```python
from build123d import *

# Parameters (mm, degrees)
EXTRUDE_1_DEPTH     = 10
SKETCH_3_W          = 10
SKETCH_3_H          = 20
EXTRUDE_2_DEPTH     = 15
EXTRUDE_3_DEPTH     = 10
EXTRUDE_4_DEPTH     = 10
SKETCH_6_W          = 10
SKETCH_6_H          = 20
EXTRUDE_5_DEPTH     = 180
SKETCH_7_W          = 10.379175533
SKETCH_7_H          = 10.878140119
SKETCH_7_W_2        = 7.174479062
SKETCH_7_H_2        = 11.599196825
CUT_EXTRUDE_1_DEPTH = 211
SKETCH_8_W          = 5
SKETCH_8_H          = 20
CUT_EXTRUDE_2_DEPTH = 25
SKETCH_9_W          = 6
SKETCH_9_H          = 16
EXTRUDE_6_DEPTH     = 10


with BuildPart() as part:
    # 草图2 → 凸台-拉伸1 (new body)
    with BuildSketch(Plane(origin=(0, 0, 0), x_dir=(1, 0, 0), z_dir=(0, 1, 0))):
        with BuildLine():
            Line((-7, 23), (7, 23))
            ThreePointArc((7, 23), (23.263455967, 16.263455967), (30, 0))
            Line((30, 0), (34, 0))
            ThreePointArc((34, 0), (26.091883092, 19.091883092), (7, 27))
            Line((7, 27), (-7, 27))
            ThreePointArc((-7, 27), (-26.091883092, 19.091883092), (-34, 0))
            Line((-34, 0), (-30, 0))
            ThreePointArc((-30, 0), (-23.263455967, 16.263455967), (-7, 23))
        make_face()
    extrude(amount=EXTRUDE_1_DEPTH)

    # 草图3 → 凸台-拉伸2 (add, symmetric)
    with BuildSketch(Plane(origin=(0, 10, 0), x_dir=(1, 0, 0), z_dir=(0, 1, 0))):
        with Locations((-35, 0)):
            Rectangle(SKETCH_3_W, SKETCH_3_H)
        with Locations((35, 0)):
            Rectangle(SKETCH_3_W, SKETCH_3_H)
    extrude(amount=EXTRUDE_2_DEPTH, both=True)

    # 草图4 → 凸台-拉伸3 (add)
    with BuildSketch(Plane(origin=(40, 0, 0), x_dir=(0, 0, -1), z_dir=(1, 0, 0))):
        with BuildLine():
            Line((-2, -5), (2, -5))
            Line((2, -5), (2, -11))
            ThreePointArc((2, -11), (0, -13), (-2, -11))
            Line((-2, -11), (-2, -5))
        make_face()
    extrude(amount=-EXTRUDE_3_DEPTH)

    # 草图5 → 凸台-拉伸4 (add)
    with BuildSketch(Plane.ZY.offset(40)):
        with BuildLine():
            Line((-2, -5), (2, -5))
            Line((2, -5), (2, -11))
            ThreePointArc((2, -11), (0, -13), (-2, -11))
            Line((-2, -11), (-2, -5))
        make_face()
    extrude(amount=-EXTRUDE_4_DEPTH)

    # 草图6 → 凸台-拉伸5 (add)
    with BuildSketch(Plane(origin=(0, 25, 0), x_dir=(1, 0, 0), z_dir=(0, 1, 0))):
        with Locations((-35, 0)):
            Rectangle(SKETCH_6_W, SKETCH_6_H)
        with Locations((35, 0)):
            Rectangle(SKETCH_6_W, SKETCH_6_H)
    extrude(amount=EXTRUDE_5_DEPTH)

    # 草图7 → 切除-拉伸1 (cut, through all)
    with BuildSketch(Plane.XZ.offset(5)):
        with Locations((-35.189587767, -15.43907006)):
            Rectangle(SKETCH_7_W, SKETCH_7_H)
        with Locations((33.587239531, -15.799598412)):
            Rectangle(SKETCH_7_W_2, SKETCH_7_H_2)
    extrude(amount=-CUT_EXTRUDE_1_DEPTH, mode=Mode.SUBTRACT)

    # 草图8 → 切除-拉伸2 (cut, symmetric)
    with BuildSketch(Plane.XZ.offset(5)):
        with Locations((-37.5, 0)):
            Rectangle(SKETCH_8_W, SKETCH_8_H)
        with Locations((37.5, 0)):
            Rectangle(SKETCH_8_W, SKETCH_8_H)
    extrude(amount=CUT_EXTRUDE_2_DEPTH, both=True, mode=Mode.SUBTRACT)

    # 草图9 → 凸台-拉伸6 (add)
    with BuildSketch(Plane.XY.offset(10)):
        with Locations((43, 28)):
            Rectangle(SKETCH_9_W, SKETCH_9_H)
        with Locations((-43, 28)):
            Rectangle(SKETCH_9_W, SKETCH_9_H)
    extrude(amount=-EXTRUDE_6_DEPTH)


solid = part.part
```
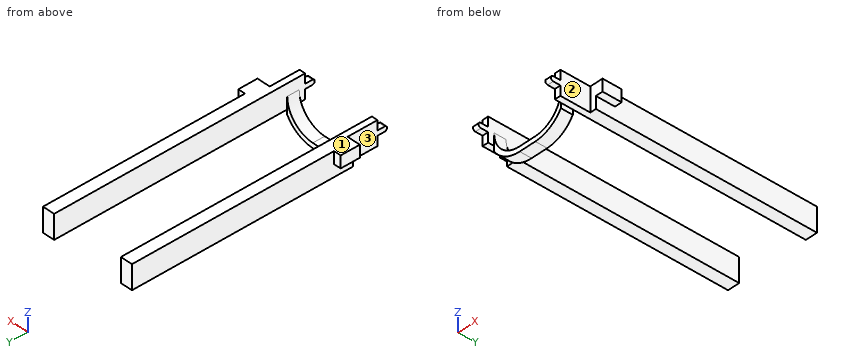
For this review, take the finished solid that the model builds, in its own axes (mm). Face numbers are marked on the shaded views. A direction names the side the tool comes from. Round coordinates to 2 decimals unless told otherwise and drop trailing zeros. Write each loop counter-clockwise with the first axis right and the second up, starting at its lowest first coordinate (ties: lowest second). Pieces come first, ordered by that corner, then holes. Notation, with made-up numbers: (65.25, 78.5) - (101.25, 78.5) arc R19 cw to (101.25, 82.5) - close; hole circle Ø9 at (69, 15.25). An arc over 180 degrees is marked (long way). Answer as CSV lines item,"result". Start each with the question number.
(1) Machinability: for the marked faces 1, 2 and 3, which of the approach directions +Z, -Z, +X, -X, +Y, -Y give a long, thin tool a straight path to every point of the face, cutting with its end or side? Answer none if there is none.
(2) For line 1 (X direction, y = 136.5, z = 8.5); line 2 (X direction, y = 25.5, z = 2); line 3 (Z direction, x = 32, y = 171), list the stretches that pass through material, from the lowest coordinate up.
(3) Add section B-B, the plane z = 7. State the section outline as (x, y) points.
(4) For pin 1 (6 mm diameter, centred on x = 8, z = -17, fed in from -Y); pin 2 (11 mm diameter, centred on x = 37, y = 91.5, fed in from -Z); pin 3 (3.5 mm diameter, centred on y = 3, z = -11.5, fed in from +X); pin 4 (2.5 mm diameter, centred on x = 32, y = -9.5, fed in from -Z), all flat-tipped, find the tip position at first contact; note any pin that passes through.
(5) Add section D-D, the plane x = 9. State the section outline as (y, z) points.
(6) Add section A-A, the plane y = 167. State the section outline as (x, z) points, plus the area to 3 significant figures.
(7) Add section C-C, the plane x = -27. State the section outline as (y, z) points, plus the area to 3 significant figures.
From the geometry:
1,face 1,"+Z, +X, -X, +Y, -Y"
1,face 2,"+Z, -Z, +X, -Y"
1,face 3,"+Z, -Z, -X, -Y"
2,line 1,"x = -40 to -30, 30 to 40"
2,line 2,"x = -46 to -30, 30 to 46"
2,line 3,"z = -10 to 10"
3,outline,"(-46, 20) - (-35, 20) - (-35, -5) - (-30, -5) - (-30, 205) - (-40, 205) - (-40, 36) - (-46, 36) - close; (30, -5) - (35, -5) - (35, 20) - (46, 20) - (46, 36) - (40, 36) - (40, 205) - (30, 205) - close"
4,pin 1,"passes through"
4,pin 2,"stops at z = -10"
4,pin 3,"stops at x = 35"
4,pin 4,"stops at z = -2"
5,outline,"(0, -26.93) - (10, -26.93) - (10, -22.91) - (0, -22.91) - close"
6,outline,"(-40, -10) - (-30, -10) - (-30, 10) - (-40, 10) - close; (30, -10) - (40, -10) - (40, 10) - (30, 10) - close"
6,area,"400 mm²"
7,outline,"(0, -18.14) - (10, -18.14) - (10, -11.36) - (0, -11.36) - close"
7,area,"67.8 mm²"
